Part model, mm, in its own coordinate system. Face numbers are marked on the shaded views. Round coordinates to 2 decimals unless told otherwise and drop trailing zeros. Loops run counter-clockwise (first coordinate to the right, second up) from the corner with the lowest first, then second, coordinate; pieces in that order, holes last.
from build123d import *

# Parameters (mm, degrees)
BOSS_EXTRUDE1_DEPTH = 3
SKETCH3_R           = 2
BOSS_EXTRUDE2_DEPTH = 5


with BuildPart() as part:
    # Sketch1 → Boss-Extrude1 (new body)
    with BuildSketch(Plane(origin=(0, 0, 0), x_dir=(1, 0, 0), z_dir=(0, 1, 0))):
        with BuildLine():
            Line((0, 0), (210, 0))
            Line((210, 0), (210, 50))
            Line((210, 50), (0, 50))
            ThreePointArc((0, 50), (-25, 25), (0, 0))
        make_face()
    extrude(amount=BOSS_EXTRUDE1_DEPTH)

    # Sketch3 → Boss-Extrude2 (add, symmetric)
    with BuildSketch(Plane.XY.offset(-25)):
        with BuildLine():
            Line((146.5, 3), (164.5, 3))
            ThreePointArc((164.5, 3), (155.5, 12), (146.5, 3))
        make_face()
        with Locations((155.5, 8)):
            Circle(SKETCH3_R, mode=Mode.SUBTRACT)
    extrude(amount=BOSS_EXTRUDE2_DEPTH, both=True)


solid = part.part
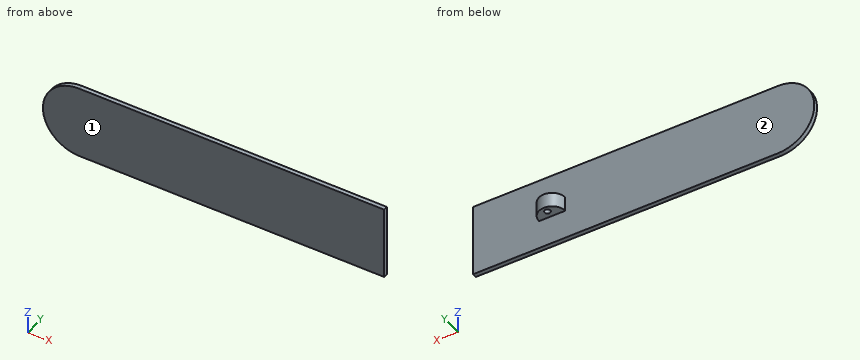
1) Slice it at B-B, the plane z = -25. Give the cut face in (x, y), then the cut area to 3 significant figures.
Values:
outline: (-25, 0) - (210, 0) - (210, 3) - (164.5, 3) arc R9 ccw to (146.5, 3) - (-25, 3) - close; hole circle Ø4 at (155.5, 8)
area: 820 mm2
2) Slice it at C-C, the plane x = 77.5. Give the cut face in (y, z).
Values:
outline: (0, -50) - (3, -50) - (3, 0) - (0, 0) - close
3) Slice it at D-D, the plane z = -12. Give the cut face in (x, y), then the cut area to 3 significant figures.
Values:
outline: (-21.35, 0) - (210, 0) - (210, 3) - (-21.35, 3) - close
area: 694 mm2
4) Drop flat-ended pins along their axis: pin 1 Ø12 at (x, z) = (108, -32) entering from -Y; pin 2 Ø1.5 at (x, y) = (40, 5) entering from +Z; pin 3 Ø4 at (x, z) = (132.5, -16) entering from +Y; pin 4 Ø2.5 at (x, y) = (155.5, 9.5) entering from +Z. Give the stop position or say it passes through.
Values:
pin 1: stops at y = 0
pin 2: passes through
pin 3: stops at y = 3
pin 4: stops at z = -20
5) Wall check: line 1 along Y through (x, z) = (155.5, -26); line 2 along Y through (x, z) = (95, -12.5); line 3 along X through (y, z) = (3.25, -21.5). Give the ranges that are in metal, low to high.
Values:
line 1: y = 0 to 6, 10 to 12
line 2: y = 0 to 3
line 3: x = 146.5 to 164.5
6) Mould opens along Y. For the marked faces 1 and 2 say: released by +Y, released by -Y, zero draft, split by the parting line, or undercut.
Values:
face 1: released by -Y
face 2: released by +Y
7) Slice it at A-A, the plane x = 155.5. Give the cut face in (y, z), then the cut area to 3 significant figures.
Values:
outline: (0, -50) - (3, -50) - (3, -30) - (6, -30) - (6, -20) - (3, -20) - (3, 0) - (0, 0) - close; (10, -30) - (12, -30) - (12, -20) - (10, -20) - close
area: 200 mm2
